from build123d import *

# Parameters (mm, degrees)
SKETCH1_W           = 35
SKETCH1_H           = 28.000000000000004
BOSS_EXTRUDE1_DEPTH = 4
SKETCH2_R           = 1.7499999999999998
CUT_EXTRUDE1_DEPTH  = 23.765104875664424
BOSS_EXTRUDE2_DEPTH = 25
CUT_EXTRUDE14_DEPTH = 66.78183639881149
SKETCH19_R          = 1.75
CUT_EXTRUDE15_DEPTH = 66.78183639881149
CUT_EXTRUDE16_DEPTH = 2.999999999999999
SKETCH21_R          = 0.49999999999999917
CUT_EXTRUDE17_DEPTH = 3.999999999999999
LPATTERN2_COUNT     = 4
LPATTERN2_PITCH     = 2
FILLET2_R           = 0.15
SKETCH22_W          = 14.999999999999995
SKETCH22_H          = 45
CUT_EXTRUDE18_DEPTH = 70.72804313904126


with BuildPart() as part:
    # Sketch1 → Boss-Extrude1 (new body)
    with BuildSketch(Plane(origin=(0, 0, 0), x_dir=(1, 0, 0), z_dir=(0, 1, 0))):
        Rectangle(SKETCH1_W, SKETCH1_H)
    extrude(amount=BOSS_EXTRUDE1_DEPTH)

    # Sketch2 → Cut-Extrude1 (cut, through all)
    with BuildSketch(Plane(origin=(0, 4, 0), x_dir=(1, 0, 0), z_dir=(0, 1, 0))):
        with Locations(Location((-7.499999999999998, -10, 0), (0, 0, 270))):
            Circle(SKETCH2_R)
        with Locations(Location((-7.499999999999998, 10, 0), (0, 0, 270))):
            Circle(SKETCH2_R)
        with Locations(Location((7.500000000000002, -10.000000000000002, 0), (0, 0, 270))):
            Circle(SKETCH2_R)
        with Locations(Location((7.500000000000002, 10, 0), (0, 0, 270))):
            Circle(SKETCH2_R)
    extrude(amount=-CUT_EXTRUDE1_DEPTH, mode=Mode.SUBTRACT)

    # Sketch3 → Boss-Extrude2 (add)
    with BuildSketch(Plane.XY.offset(14)):
        Polygon((-17.499999999999996, 4), (17.500000000000004, 4), (17.50000000000001, -46), (-17.499999999999993, -46), align=None)
    extrude(amount=BOSS_EXTRUDE2_DEPTH)

    # Sketch18 → Cut-Extrude14 (cut, through all)
    with BuildSketch(Plane(origin=(0, 4, 0), x_dir=(1, 0, 0), z_dir=(0, 1, 0))):
        Polygon((-17.499999999999996, -9.999999999999998), (-10.499999999999998, -10.000000000000002), (-10.499999999999998, -11.500000000000002), (-17.499999999999996, -11.500000000000004), align=None)
        Polygon((17.500000000000004, 10.000000000000002), (10.500000000000002, 10), (10.500000000000002, 11.5), (17.500000000000004, 11.500000000000004), align=None)
    extrude(amount=-CUT_EXTRUDE14_DEPTH, mode=Mode.SUBTRACT)

    # Sketch19 → Cut-Extrude15 (cut, through all)
    with BuildSketch(Plane(origin=(0, 4, 0), x_dir=(1, 0, 0), z_dir=(0, 1, 0))):
        with Locations(Location((-7.499999999999998, 0, 0), (0, 0, 270))):
            Circle(SKETCH19_R)
        with Locations(Location((7.500000000000005, 0, 0), (0, 0, 270))):
            Circle(SKETCH19_R)
    extrude(amount=-CUT_EXTRUDE15_DEPTH, mode=Mode.SUBTRACT)

    # Sketch20 → Cut-Extrude16 (cut)
    with BuildSketch(Plane.XZ):
        Polygon((10.96410161513776, 9.3e-16), (9.23205080756888, 2.9999999999999996), (5.767949192431128, 2.9999999999999987), (4.035898384862253, -1.5e-16), (5.767949192431131, -3), (9.232050807568884, -2.9999999999999996), align=None)
        Polygon((-10.964101615137752, 5.88e-15), (-9.232050807568879, -2.999999999999999), (-5.767949192431124, -3.000000000000003), (-4.035898384862242, -3.87e-15), (-5.7679491924311215, 3.000000000000001), (-9.232050807568873, 3.0000000000000053), align=None)
    extrude(amount=-CUT_EXTRUDE16_DEPTH, mode=Mode.SUBTRACT)

    # Sketch21 → Cut-Extrude17 (cut)
    with BuildSketch(Plane(origin=(0, 4, 0), x_dir=(1, 0, 0), z_dir=(0, 1, 0))):
        with Locations((-16.999999999999996, -10.000000000000002)):
            Circle(SKETCH21_R)
    cut_extrude17 = extrude(amount=-CUT_EXTRUDE17_DEPTH, mode=Mode.SUBTRACT)

    # LPattern2: Cut-Extrude17 ×4
    with Locations(*[(i * LPATTERN2_PITCH, 0, 0) for i in range(1, LPATTERN2_COUNT)]):
        add(cut_extrude17, mode=Mode.SUBTRACT)

    # Fillet2
    fillet2_edges = [part.edges().sort_by_distance(p)[0] for p in [
        (-16.499999999999996, 2.0000000000000004, 10.000000000000002),
        (-12.499999999999996, 2.0000000000000004, 10.000000000000005),
        (-13.499999999999996, 2, 10),
        (-14.499999999999996, 2.0000000000000004, 10.000000000000004),
        (-15.499999999999996, 2, 10),
        (-11.499999999999996, 2, 10.000000000000002),
        (-17.499999999999996, 2, 9.999999999999998),
    ]]
    fillet(fillet2_edges, radius=FILLET2_R)

    # Sketch22 → Cut-Extrude18 (cut, through all)
    with BuildSketch(Plane.ZY.offset(17.499999999999996)):
        with Locations((21.5, -23.5)):
            Rectangle(SKETCH22_W, SKETCH22_H)
    extrude(amount=-CUT_EXTRUDE18_DEPTH, mode=Mode.SUBTRACT)


solid = part.part
CAD build for the part. Positions are in the model's coordinates, mm. A direction names the side the tool comes from. Give positions to 0.01 mm unless a question says otherwise; leave off trailing zeros. Loops run counter-clockwise (first coordinate to the right, second up) from the corner with the lowest first, then second, coordinate; pieces in that order, holes last. Notation, with made-up numbers: M 61.25,-26.5 L 76.25,-26.5 A21 ccw 76.25,-6.5 Z; hole C 3.5,-8.75 d5. An arc over 180 degrees is marked long. Answer in a Markdown table with one row per item. Add a question column.
Item 1: Tool access for faces 4 (the face through (10.5, 2, -11)), 5 (the face through (9, 3, 1.4)), 6 (the face through (0, -24, 29)), 7 (the face through (-14, 2, 11.5)): list every direction of +Z, -Z, +X, -X, +Y, -Y with a clear straight run to the whole face (end or side of a thin tool).
Item 2: Band-saw the part on C-C on z = 6. Give the cut face in (x, y).
Item 3: Band-saw the part on A-A on x = -7.5. Give the cut face in (y, z), then the cut area to 4 significant figures.
Item 4: Mould opens along Z. For faces 1 (the face through (0, 2, -14)), 2 (the face through (17.5, -13, 31)), 3 (the face through (4.9, 1.5, 1.5)) say: +Z half, -Z half, draft (parallel to the pull), parting line (faces both ways), or undercut.
Item 5: Band-saw the part on B-B on x = 1. Give the cut face in (y, z).
Item 6: Drop flat-ended pins along their axis: P1, Ø2, axis at x = 11, y = -27, coming from the -Z side; P2, Ø3, axis at x = -7.5, z = -10, coming from the +Y side; P3, Ø1.8, axis at x = 7.5, z = 1, coming from the -Y side; P4, Ø6.5, axis at x = -8.5, z = 0, coming from the -Y side. Give the stop position or say it passes through.
Item 7: Probe probe 1 along Z at (x, y) = (-7, 1); probe 2 along Y at (x, z) = (-5, 10); probe 3 along Z at (x, y) = (2, -42.5). List the from-to ranges inside material, lowest first.
Item 8: Band-saw the part on D-D on y = -27.5. Give the cut face in (x, z).
Reply:
| question | item | result |
|---|---|---|
| 1 | face 4 | +X, +Y, -Y |
| 1 | face 5 | -Y |
| 1 | face 6 | -Z, +X, -X, -Y |
| 1 | face 7 | -X, +Y, -Y |
| 2 | outline | M -17.5,0 L 17.5,0 L 17.5,4 L -17.5,4 Z |
| 3 | outline | M -46,29 L -1,29 L -1,14 L 0,14 L 0,11.75 L 4,11.75 L 4,39 L -46,39 Z; M 0,-14 L 4,-14 L 4,-11.75 L 0,-11.75 Z; M 0,-8.25 L 4,-8.25 L 4,-1.75 L 3,-1.75 L 3,-3 L 0,-3 Z; M 0,3 L 3,3 L 3,1.75 L 4,1.75 L 4,8.25 L 0,8.25 Z |
| 3 | area | 637.5 mm^2 |
| 4 | face 1 | -Z half |
| 4 | face 2 | draft |
| 4 | face 3 | undercut |
| 5 | outline | M -46,29 L -1,29 L -1,14 L 0,14 L 0,-14 L 4,-14 L 4,39 L -46,39 Z |
| 6 | P1 | stops at z = 29 |
| 6 | P2 | passes through |
| 6 | P3 | stops at y = 3 |
| 6 | P4 | stops at y = 0 |
| 7 | probe 1 | z = -14 to -11.68, -8.32 to -3, 3 to 8.32, 11.68 to 39 |
| 7 | probe 2 | y = 0 to 4 |
| 7 | probe 3 | z = 29 to 39 |
| 8 | outline | M -17.5,29 L 17.5,29 L 17.5,39 L -17.5,39 Z |
